from build123d import *

# Parameters (mm, degrees)
SKETCH1_W           = 14
SKETCH1_H           = 9
SKETCH1_R           = 2.5
BOSS_EXTRUDE1_DEPTH = 3
FILLET1_R           = 0.5
BOSS_EXTRUDE2_DEPTH = 2
FILLET2_R           = 0.1


with BuildPart() as part:
    # Sketch1 → Boss-Extrude1 (new body)
    with BuildSketch(Plane.XY):
        Rectangle(SKETCH1_W, SKETCH1_H)
        Circle(SKETCH1_R, mode=Mode.SUBTRACT)
    extrude(amount=BOSS_EXTRUDE1_DEPTH)

    # Fillet1
    fillet1_edges = [part.edges().sort_by_distance(p)[0] for p in [
        (-7, 4.5, 1.5),
        (7, 4.5, 1.5),
        (7, -4.5, 1.5),
        (-7, -4.5, 1.5),
    ]]
    fillet(fillet1_edges, radius=FILLET1_R)

    # Sketch2 → Boss-Extrude2 (add)
    with BuildSketch(Plane.XY.offset(3)):
        with BuildLine():
            Line((-5.028169014, -0.852945699), (-7, -1.187434209))
            ThreePointArc((-7, -1.187434209), (-6.461781127, -2.942003512), (-5.491812087, -4.5))
            Line((-5.491812087, -4.5), (-3.944822767, -3.232394366))
            ThreePointArc((-3.944822767, -3.232394366), (-4.641561091, -2.113270128), (-5.028169014, -0.852945699))
        make_face()
        with BuildLine():
            Line((5.491812087, 4.5), (3.944822767, 3.232394366))
            ThreePointArc((3.944822767, 3.232394366), (4.641561091, 2.113270128), (5.028169014, 0.852945699))
            Line((5.028169014, 0.852945699), (7, 1.187434209))
            ThreePointArc((7, 1.187434209), (6.461781127, 2.942003512), (5.491812087, 4.5))
        make_face()
    extrude(amount=BOSS_EXTRUDE2_DEPTH)

    # Fillet2
    fillet2_edges = [part.edges().sort_by_distance(p)[0] for p in [
        (-5.028169014, -0.852945699, 4),
        (-7, -1.187434209, 4),
        (-5.491812087, -4.5, 4),
        (-4.641561091, -2.113270128, 5),
        (-3.944822767, -3.232394366, 4),
        (-6.014084507, -1.020189954, 5),
        (-6.461781127, -2.942003512, 5),
        (-4.718317427, -3.866197183, 5),
        (5.491812087, 4.5, 4),
        (3.944822767, 3.232394366, 4),
        (6.014084507, 1.020189954, 5),
        (5.028169014, 0.852945699, 4),
        (6.461781127, 2.942003512, 5),
        (7, 1.187434209, 4),
        (4.718317427, 3.866197183, 5),
        (4.641561091, 2.113270128, 5),
    ]]
    fillet(fillet2_edges, radius=FILLET2_R)


solid = part.part
Can you work these out from the model? Positions are in its coordinate system, mm. A direction names the side the tool comes from. Give positions to 0.01 mm unless a question says otherwise; leave off trailing zeros. Loops run counter-clockwise (first coordinate to the right, second up) from the corner with the lowest first, then second, coordinate; pieces in that order, holes last. Notation, with made-up numbers: (-11.5, 50.25) -> (38.5, 50.25) arc R26 cw to (38.5, 78.25) -> close; hole circle Ø6 at (70, -7.5). An arc over 180 degrees is marked (long way). Use one line per item in the form item = value.
1) If we section it at A-A (z = 3.85): Please give me the cut outline in (x, y), plus the area to 3 significant figures.
Answers:
outline = (-6.98, -1.29) arc R7.1 ccw to (-5.56, -4.42) arc R0.1 ccw to (-5.41, -4.44) -> (-4.02, -3.3) arc R0.1 ccw to (-4.01, -3.16) arc R5.1 cw to (-5.01, -0.95) arc R0.1 ccw to (-5.13, -0.87) -> (-6.9, -1.17) arc R0.1 ccw to start; (4.01, 3.16) arc R5.1 cw to (5.01, 0.95) arc R0.1 ccw to (5.13, 0.87) -> (6.9, 1.17) arc R0.1 ccw to (6.98, 1.29) arc R7.1 ccw to (5.56, 4.42) arc R0.1 ccw to (5.41, 4.44) -> (4.02, 3.3) arc R0.1 ccw to start
area = 12.6 mm²
2) I need wall thicknesses on line 1 along Y through (x, z) = (0, 1); line 2 along Z through (x, y) = (5.5, -1.5); line 3 along X through (y, z) = (0.25, 1.9). Which ranges of each line are inside material? Lowest first, please.
Answers:
line_1 = -4.5 to -2.5, 2.5 to 4.5
line_2 = 0 to 3
line_3 = -7 to -2.49, 2.49 to 7
3) Will this pin go through, and if not, where does the flat tip stop? pin 1 (1.5 mm diameter, centred on x = -4, y = 1.5, fed in from +Z).
Answers:
pin_1 = 3
4) If we section it at C-C (y = 0): Please give me the cut outline in (x, z).
Answers:
outline = (-7, 0) -> (-2.5, 0) -> (-2.5, 3) -> (-7, 3) -> close; (2.5, 0) -> (7, 0) -> (7, 3) -> (2.5, 3) -> close
5) For faces 1 (the face through (-4.727, -3.874, 3.937)), 2 (the face through (-2, 2, 3)), 3 (the face through (-4.634, -2.129, 3.937)), which set-ups out of +Z, -Z, +X, -X, +Y, -Y let a thin tool reach every point of the face, with its end or its side?
Answers:
face_1 = +Z, +X, -Y
face_2 = +Z
face_3 = +Z, +X, +Y
6) If we section it at D-D (z = 2): Please give me the cut outline in (x, y).
Answers:
outline = (-7, -4) arc R0.5 ccw to (-6.5, -4.5) -> (6.5, -4.5) arc R0.5 ccw to (7, -4) -> (7, 4) arc R0.5 ccw to (6.5, 4.5) -> (-6.5, 4.5) arc R0.5 ccw to (-7, 4) -> close; hole circle Ø5 at (0, 0)
7) We'd pull the mould along Y, two halves only. Please class faces 4 (the face through (-0.54, -2.44, 1.48)), 5 (the face through (-7, 0, 1)), 6 (the face through (-6.47, -2.92, 3.94)), 7 (the face through (-6.001, -1.018, 3.937)): released by +Y, released by -Y, zero draft, split by the parting line, or undercut.
Answers:
face_4 = undercut
face_5 = zero draft
face_6 = released by -Y
face_7 = released by +Y
8) If we section it at B-B (x = 0): Please give me the cut outline in (y, z), plus the area to 3 significant figures.
Answers:
outline = (-4.5, 0) -> (-2.5, 0) -> (-2.5, 3) -> (-4.5, 3) -> close; (2.5, 0) -> (4.5, 0) -> (4.5, 3) -> (2.5, 3) -> close
area = 12.0 mm²
